```python
from build123d import *

# Parameters (mm, degrees)
F4_R     = 5
F5_DEPTH = 2.5
F6_DEPTH = 2.5


with BuildPart() as f2:
    # F2: sweep along a path in F1
    with BuildLine(Plane.YZ) as f2_path:
        Line((0, -20), (90, -20))
        ThreePointArc((90, -20), (97.071068, -22.928932), (100, -30))
        Line((100, -30), (100, -80))
        Line((100, -80), (100, -130))
        ThreePointArc((100, -130), (97.071068, -137.071068), (90, -140))
        Line((90, -140), (0, -140))
    # F0 (on Front) → F2 (sweep)
    with BuildSketch(Plane.XZ):
        with BuildLine():
            Line((2.5, -12), (2.5, 0))
            Line((2.5, 0), (2.5, 12))
            ThreePointArc((2.5, 12), (3.37868, 14.12132), (5.5, 15))
            Line((5.5, 15), (10, 15))
            Line((10, 15), (10, 20))
            Line((10, 20), (0, 20))
            Line((0, 20), (-10, 20))
            Line((-10, 20), (-10, 15))
            Line((-10, 15), (-5.5, 15))
            ThreePointArc((-5.5, 15), (-3.37868, 14.12132), (-2.5, 12))
            Line((-2.5, 12), (-2.5, 0))
            Line((-2.5, 0), (-2.5, -12))
            ThreePointArc((-2.5, -12), (-3.37868, -14.12132), (-5.5, -15))
            Line((-5.5, -15), (-10, -15))
            Line((-10, -15), (-10, -20))
            Line((-10, -20), (0, -20))
            Line((0, -20), (10, -20))
            Line((10, -20), (10, -15))
            Line((10, -15), (5.5, -15))
            ThreePointArc((5.5, -15), (3.37868, -14.12132), (2.5, -12))
        make_face()
    sweep(path=f2_path.line)

    # F4 (on Right) → F5 (join, symmetric)
    with BuildSketch(Plane.YZ):
        with BuildLine():
            Line((0, 50), (0, 20))
            Line((0, 20), (70, 20))
            Line((70, 20), (35.548045, 62.580075))
            ThreePointArc((35.548045, 62.580075), (13.327703, 68.854189), (0, 50))
        make_face()
        with Locations((20, 50)):
            Circle(F4_R, mode=Mode.SUBTRACT)
    extrude(amount=F5_DEPTH, both=True)

    # F4 (on Right) → F6 (join, symmetric)
    with BuildSketch(Plane.YZ):
        with BuildLine():
            Line((0, 50), (0, 20))
            Line((0, 20), (70, 20))
            Line((70, 20), (35.548045, 62.580075))
            ThreePointArc((35.548045, 62.580075), (13.327703, 68.854189), (0, 50))
        make_face()
        with Locations((20, 50)):
            Circle(F4_R, mode=Mode.SUBTRACT)
        with BuildLine():
            Line((35.548045, -222.580075), (70, -180))
            Line((70, -180), (0, -180))
            Line((0, -180), (0, -210))
            ThreePointArc((0, -210), (13.327703, -228.854189), (35.548045, -222.580075))
        make_face()
        with Locations((20, -210)):
            Circle(F4_R, mode=Mode.SUBTRACT)
    extrude(amount=F6_DEPTH, both=True)


solid = f2.part
```
CAD build for the part. Positions are in the model's coordinates, mm. A direction names the side the tool comes from. Coordinates: 2 decimals unless noted, no trailing zeros. Write each loop counter-clockwise with the first axis right and the second up, starting at its lowest first coordinate (ties: lowest second). Pieces come first, ordered by that corner, then holes. Notation, with made-up numbers: (0.5, -11.5) -> (26.5, -11.5) arc R19 ccw to (26.5, 1.5) -> close; hole circle Ø4 at (-19.75, 66.5). An arc over 180 degrees is marked (long way). Return JSON: item names as keys, results as strings. Group by question number.
Q1. Which spindle directions (+Z, -Z, +X, -X, +Y, -Y) get a long thin tool onto all of the face, cutting with end or side? Do faces 4 (the face through (-2.5, 27, -199)), 5 (the face through (0.14, 96.99, -22.85)), 6 (the face through (-7.719, 122.168, -161.468)), 7 (the face through (0, 0, 8)), 8 (the face through (7.72, 100.49, -19.28)). Say none if no direction does.
Q2. Cut at B-B, the plane z = -195.5. Give the cut face in (x, y).
Q3. Cut at A-A, the plane y = 20. State how many separate pieces and enclosed holes the cut face has, then the cut area to 3 significant figures.
Q4. Pull direction Z, two halves, no side cores. Call faces 1 (the face through (-7.78, 100.49, -19.28)), 2 (the face through (10, 138, -80)), 3 (the face through (0.04, 52.53, -201.59)): released by +Z, released by -Z, zero draft, split by the parting line, or undercut.
Q5. Flat gauge pins, fed straight in: pin 1 (2 mm diameter, centred on x = -2, y = 116, fed in from -Z); pin 2 (3.5 mm diameter, centred on x = -7, y = 49, fed in from -Z); pin 3 (2 mm diameter, centred on x = 8, y = 23.5, fed in from +Z). Where does each tip first touch, or does it go through?
Q6. Drill centre lines: line 1 (Z direction, x = -0.6, y = 20); line 2 (Z direction, x = -6.25, y = 75.5); line 3 (Y direction, x = -6.75, z = -63). Where is each one in solid material? Low to high.
Returned:
{
 "1": {"face 4": "-Z, -X, +Y, -Y", "face 5": "+X, -X, -Y", "face 6": "-X", "face 7": "+Z, -Z, +X, -X, -Y", "face 8": "+X"},
 "2": {"outline": "(-2.5, 0) -> (2.5, 0) -> (2.5, 57.46) -> (-2.5, 57.46) -> close"},
 "3": {"separate pieces": "4", "enclosed holes": "0", "area": "1,120 mm2"},
 "4": {"face 1": "undercut", "face 2": "zero draft", "face 3": "released by -Z"},
 "5": {"pin 1": "stops at z = -173.3", "pin 2": "stops at z = -180", "pin 3": "stops at z = 20"},
 "6": {"line 1": "z = -230 to -215, -205 to -140, -20 to 45, 55 to 70", "line 2": "z = -180 to -175, -145 to -140, -20 to -15, 15 to 20", "line 3": "y = 100 to 105, 135 to 140"}
}
